Study the drawing (mm; zero at the part's minimum x, y, z) and answer. A direction names the side the tool comes from. Give positions to 0.01 mm unless a question says otherwise; leave off trailing zeros. Write each loop counter-clockwise with the first axis right and the second up, starting at its lowest first coordinate (ties: lowest second). Pieces come first, ordered by that corner, then holes. Notation, with made-up numbers: (70, 61) - (94, 61) arc R25 ccw to (94, 93) - close; hole circle Ø3 at (38, 49). An arc over 180 degrees is marked (long way). One line per item, written item: value. Start each with the question number.
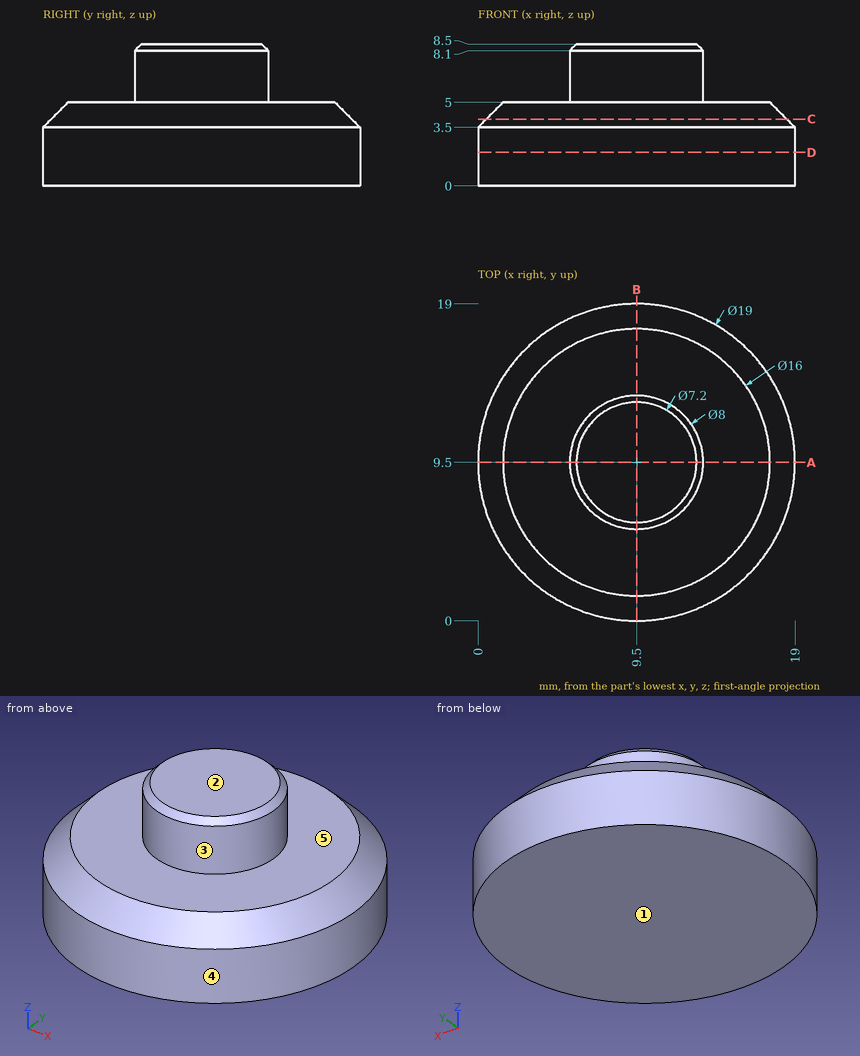
Item 1: Each of these flat-tipped pins is pushed along its axis until it touches: pin 1 Ø2 at (x, z) = (13.5, 7.5) entering from -Y; pin 2 Ø4 at (x, y) = (16, 6.5) entering from +Z; pin 3 Ø1 at (x, z) = (3.5, 4.5) entering from -Y. Where does it stop, or does it pass through?
Item 2: The mould has two halves that part along Z. Classify the marked faces 1, 2 and 3: +Z half, -Z half, draft (parallel to the pull), parting line (faces both ways), or undercut.
Item 3: Find section D-D on z = 2. Determine the outline of the cut face in (x, y), plus the area to 3 significant figures.
Item 4: For the marked faces 4 and 5, determine the directions among +Z, -Z, +X, -X, +Y, -Y from which every point of the face is accessible in a straight line to the end or side of a thin tool.
Item 5: Find section C-C on z = 4. Determine the outline of the cut face in (x, y), plus the area to 3 significant figures.
Item 6: Straight lines are drawn through the part: line 1 along Z through (x, y) = (5.5, 15.25); line 2 along Z through (x, y) = (7.25, 12.75); line 3 along X through (y, z) = (10.25, 5.25). For each, find the intervals that lie inside material, in ascending order.
Item 7: Find section A-A on y = 9.5. Determine the outline of the cut face in (x, z), plus the area to 3 significant figures.
Values:
1. pin 1: y = 6.85
1. pin 2: z = 5
1. pin 3: y = 2.66
2. face 1: -Z half
2. face 2: +Z half
2. face 3: draft
3. outline: circle Ø19 at (9.5, 9.5)
3. area: 284 mm^2
4. face 4: +Z, -Z
4. face 5: +Z
5. outline: circle Ø18 at (9.5, 9.5)
5. area: 254 mm^2
6. line 1: 0 to 5
6. line 2: 0 to 8.15
6. line 3: 5.57 to 13.43
7. outline: (0, 0) - (19, 0) - (19, 3.5) - (17.5, 5) - (13.5, 5) - (13.5, 8.1) - (13.1, 8.5) - (5.9, 8.5) - (5.5, 8.1) - (5.5, 5) - (1.5, 5) - (0, 3.5) - close
7. area: 121 mm^2
